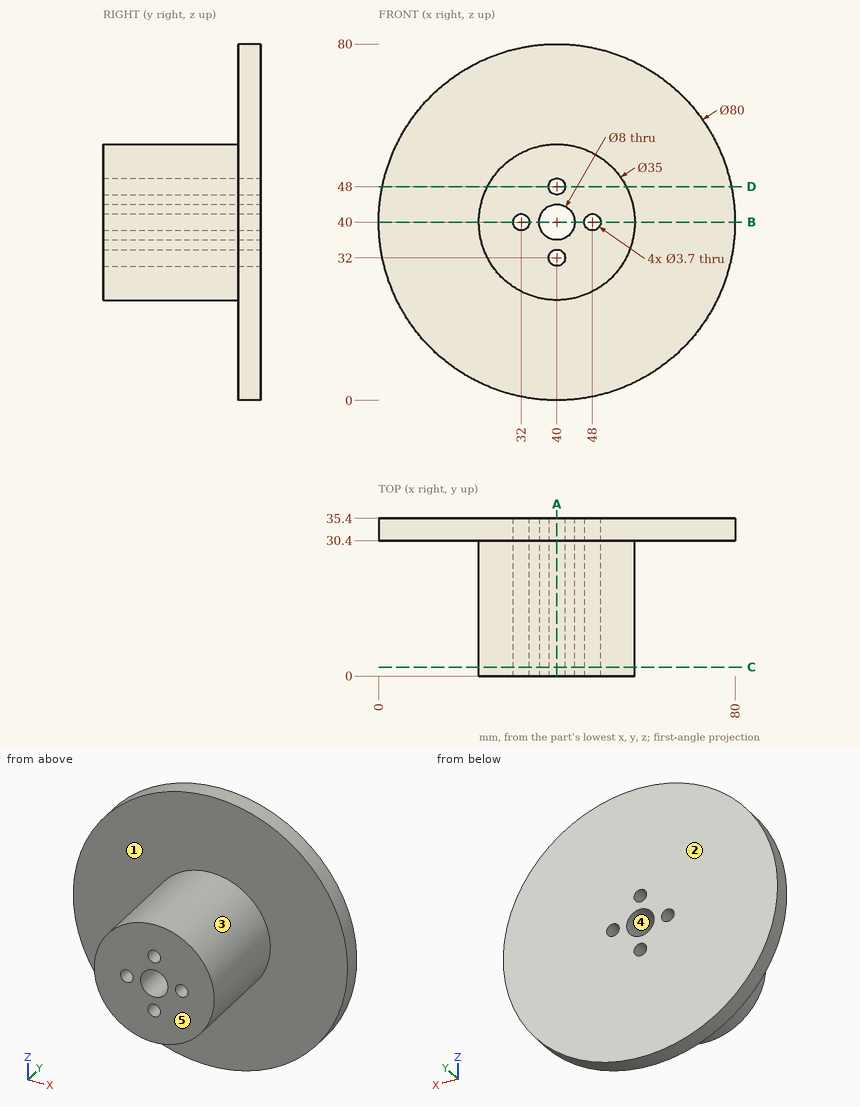
Here's the drawing with two shaded views (mm, measured from the low corner). I have some questions. A direction names the side the tool comes from. Round coordinates to 2 decimals unless told otherwise and drop trailing zeros. Loops run counter-clockwise (first coordinate to the right, second up) from the corner with the lowest first, then second, coordinate; pieces in that order, holes last. Notation, with made-up numbers: M 46,2.5 L 94,2.5 A27 cw 94,32.5 Z; hole C -8,-38 d11. An arc over 180 degrees is marked long. Put each result on its own line as item: value.
Q1. I need wall thicknesses on probe 1 along X at (y, z) = (28, 38); probe 2 along X at (y, z) = (31, 38); probe 3 along Y at (x, z) = (71.5, 38.5). Which ranges of each line are inside material? Lowest first, please.
Check result:
probe 1: 22.61 to 36.54, 43.46 to 57.39
probe 2: 0.05 to 36.54, 43.46 to 79.95
probe 3: 30.4 to 35.4
Q2. Imagine slicing it at D-D (z = 48). Write out the boundary of the cut face in (x, y).
Check result:
outline: M 0.81,30.4 L 24.44,30.4 L 24.44,0 L 38.15,0 L 38.15,35.4 L 0.81,35.4 Z; M 41.85,0 L 55.56,0 L 55.56,30.4 L 79.19,30.4 L 79.19,35.4 L 41.85,35.4 Z
Q3. Thinking about a two-plate mould opening in Z: for the marked faces 3, 4 and 5, which applies, released by +Z, released by -Z, zero draft, split by the parting line, or undercut?
Check result:
face 3: split by the parting line
face 4: undercut
face 5: zero draft
Q4. Imagine slicing it at C-C (y = 2). Write out the boundary of the cut face in (x, z), then the cut area to 3 significant figures.
Check result:
outline: C 40,40 d35; hole C 32,40 d3.7; hole C 40,40 d8; hole C 40,32 d3.7; hole C 40,48 d3.7; hole C 48,40 d3.7
area: 869 mm2
Q5. Imagine slicing it at A-A (x = 40). Write out the boundary of the cut face in (y, z).
Check result:
outline: M 0,22.5 L 30.4,22.5 L 30.4,0 L 35.4,0 L 35.4,30.15 L 0,30.15 Z; M 0,33.85 L 35.4,33.85 L 35.4,36 L 0,36 Z; M 0,44 L 35.4,44 L 35.4,46.15 L 0,46.15 Z; M 0,49.85 L 35.4,49.85 L 35.4,80 L 30.4,80 L 30.4,57.5 L 0,57.5 Z
Q6. On a 3-axis mill with a long thin cutter (end or side, diameter ignored), from which of +Z, -Z, +X, -X, +Y, -Y can I reach the whole of each face in a straight line? I mean the marked faces 1 and 2. Say none if no direction works.
Check result:
face 1: -Y
face 2: +Z, -Z, +X, -X, +Y
Q7. For pin 1 (6 mm diameter, centred on x = 38, y = 24, fed in from +Z); pin 2 (10 mm diameter, centred on y = 20.5, z = 32, fed in from -X); pin 3 (3.5 mm diameter, centred on x = 40, z = 48, fed in from -Y); pin 4 (1.5 mm diameter, centred on x = 68, z = 50, fed in from -Y), each with a flat end and sliding along its axis, tell me the tip position at first contact or that it passes through.
Check result:
pin 1: z = 57.5
pin 2: x = 22.76
pin 3: through
pin 4: y = 30.4
Q8. Imagine slicing it at B-B (z = 40). Write out the boundary of the cut face in (x, y).
Check result:
outline: M 0,30.4 L 22.5,30.4 L 22.5,0 L 30.15,0 L 30.15,35.4 L 0,35.4 Z; M 33.85,0 L 36,0 L 36,35.4 L 33.85,35.4 Z; M 44,0 L 46.15,0 L 46.15,35.4 L 44,35.4 Z; M 49.85,0 L 57.5,0 L 57.5,30.4 L 80,30.4 L 80,35.4 L 49.85,35.4 Z
